Design review of the part built by this model. Coordinates are the model's own, in mm. Face numbers are marked on the shaded views. A direction names the side the tool comes from. Give positions to 0.01 mm unless a question says otherwise; leave off trailing zeros. Order: outer loops, then holes, each group sorted by start corner. A loop starts at its lowest first (then second) coordinate and runs counter-clockwise, first axis right, second up. Notation, with made-up numbers: M -28,20 L -8,20 A15 ccw -8,34 Z; hole C -16.5,22.25 d2. An arc over 180 degrees is marked long. Put each result on its own line as item: value. Start each with the question number.
Autodesk Inventor part; units mm, degrees
ref_plane "YZ Plane" through (0, 0, 0) normal (1, 0, 0) x (0, 1, 0)
ref_plane "XZ Plane" through (0, 0, 0) normal (0, 1, 0) x (-1, 0, 0)
ref_plane "XY Plane" through (0, 0, 0) normal (0, 0, 1) x (1, 0, 0)
sketch "Sketch1" plane through (0, 0, 0) normal (0, 1, 0) x (-1, 0, 0)
  line L0 (0, 0) -> (67, 0)
  line L1 (67, 0) -> (67, -91.44)
  line L2 (67, -91.44) -> (0, -91.44)
  line L3 (0, -91.44) -> (0, 0)
  dimension "d0" = 91.44
  dimension "d1" = 67
extrude "Extrusion1" add sketch "Sketch1" along normal blind 3.81
sketch "Sketch3" plane through (0, 3.81, 0) normal (0, 1, 0) x (1, 0, 0)
  line L0 (-67, 0) -> (0, 0)
  line L1 (0, 91.44) -> (-67, 91.44)
  line L2 (-67, 0) -> (-59.535, 0)
  line L3 (-62.555, 4.445) -> (-62.555, 86.995)
  line L4 (-62.555, 91.44) -> (-67, 91.44)
  line L5 (-67, 91.44) -> (-67, 0)
  line L6 (-33.5, 0) -> (-33.5, 91.44) construction
  line L7 (-59.535, 0) -> (-33.5, 0)
  line L8 (-33.5, 4.445) -> (-62.555, 4.445)
  line L9 (-62.555, 91.44) -> (-33.5, 91.44)
  line L10 (-33.5, 86.995) -> (-62.555, 86.995)
  line L11 (0, 0) -> (-67, 0)
  line L12 (0, 0) -> (-7.465, 0)
  line L13 (-4.445, 4.445) -> (-4.445, 86.995)
  line L14 (-4.445, 91.44) -> (0, 91.44)
  line L15 (0, 91.44) -> (0, 0)
  line L16 (-33.5, 4.445) -> (-4.445, 4.445)
  line L17 (-4.445, 91.44) -> (-33.5, 91.44)
  line L18 (-33.5, 86.995) -> (-4.445, 86.995)
  dimension "d25" = 4.445
  dimension "d27" = 4.445
  dimension "d28" = 4.445
  dimension "d30" = 26.035
  dimension "d31" = 4.445
  dimension "d32" = 86.995
  dimension "d33" = 4.445
extrude "Extrusion2" add sketch "Sketch3" along normal blind 39
fillet "Fillet1" radius 3.175 4 edges at (-67, 21.405, -91.44) (-67, 21.405, 0) (0, 21.405, 0) (0, 21.405, -91.44)
properties part number "Case RevA"
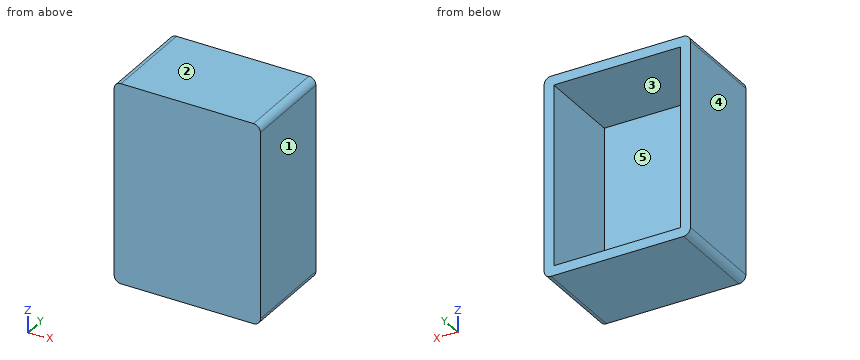
1. The part is to be moulded in two halves that separate along X. For the marked faces 1, 2 and 3, say which applies: +X half, -X half, draft (parallel to the pull), parting line (faces both ways), or undercut.
2. Consider section B-B on x = -8. Give the boundary of the cut face in (y, z) (3 decimals).
3. Insertion check: pin 1 (12 mm diameter, centred on x = -12.5, z = -28, fed in from +Y). The pin has a flat end and moves straight along its axis. Give the tip position at first contact, or say it passes through.
4. Consider section A-A on y = 15. Give the boundary of the cut face in (x, z) (3 decimals), then the cut area to 3 significant figures.
5. To check wall thickness, follow probe 1 along X at (y, z) = (34.5, -52.5) (3 decimals); probe 2 along Z at (x, y) = (-55, 22.5) (3 decimals); probe 3 along Y at (x, z) = (-58, -51). State the ranges of each line that lie inside material, in increasing order.
6. Consider section C-C on z = -81.5. Give the boundary of the cut face in (x, y) (3 decimals), then the cut area to 3 significant figures.
7. Machinability: for the marked faces 4 and 5, which of the approach directions +Z, -Z, +X, -X, +Y, -Y give a long, thin tool a straight path to every point of the face, cutting with its end or side? Answer none if there is none.
Returned:
1. face 1: +X half
1. face 2: draft
1. face 3: undercut
2. outline: M 0,-91.44 L 42.81,-91.44 L 42.81,-86.995 L 3.81,-86.995 L 3.81,-4.445 L 42.81,-4.445 L 42.81,0 L 0,0 Z
3. pin 1: stops at y = 3.81
4. outline: M -67,-88.265 A3.175 ccw -63.825,-91.44 L -3.175,-91.44 A3.175 ccw 0,-88.265 L 0,-3.175 A3.175 ccw -3.175,0 L -63.825,0 A3.175 ccw -67,-3.175 Z; hole M -62.555,-86.995 L -4.445,-86.995 L -4.445,-4.445 L -62.555,-4.445 Z
4. area: 1,320 mm2
5. probe 1: x = -67 to -62.555, -4.445 to 0
5. probe 2: z = -91.44 to -86.995, -4.445 to 0
5. probe 3: y = 0 to 3.81
6. outline: M -67,0 L 0,0 L 0,42.81 L -4.445,42.81 L -4.445,3.81 L -62.555,3.81 L -62.555,42.81 L -67,42.81 Z
6. area: 602 mm2
7. face 4: +Z, -Z, -X, +Y, -Y
7. face 5: +Y
